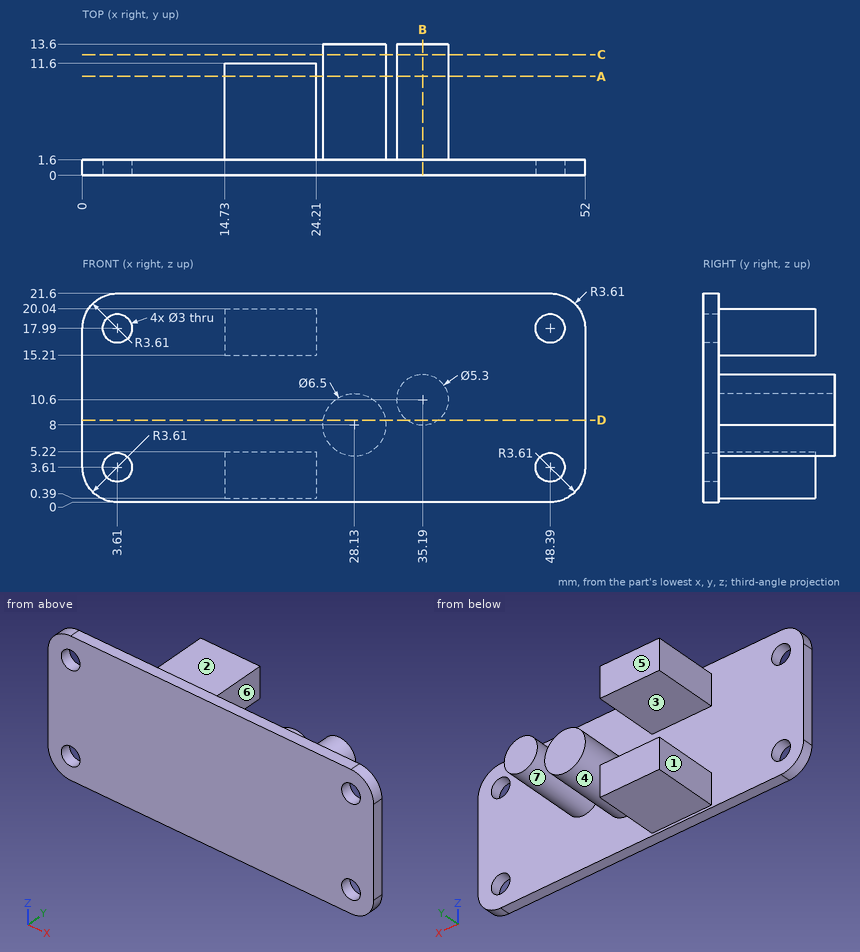
Can you work these out from the drawing? Everything is in mm from the part's minimum corner. A direction names the side the tool comes from. Round coordinates to 2 decimals unless told otherwise and drop trailing zeros. Loops run counter-clockwise (first coordinate to the right, second up) from the corner with the lowest first, then second, coordinate; pieces in that order, holes last. Notation, with made-up numbers: (-2.5, 53) - (13.5, 53) arc R24 ccw to (13.5, 80) - close; hole circle Ø7 at (70, -37). An arc over 180 degrees is marked (long way). Answer in a Markdown table with one row per item. Add a question column.
(1) If we section it at D-D (z = 8.5): Please give me the cut outline in (x, y), plus the area to 3 significant figures.
(2) For the marked faces 1, 2, 3 and 4, which set-ups out of +Z, -Z, +X, -X, +Y, -Y let a thin tool reach every point of the face, with its end or its side?
(3) I need wall thicknesses on line 1 along X through (y, z) = (8, 1.25); line 2 along Y through (x, z) = (26, 12.25); line 3 along Z through (x, y) = (35, 10.5). Which ranges of each line are inside material? Lowest first, please.
(4) If we section it at C-C (y = 12.5): Please give me the cut outline in (x, z).
(5) I'm going to push flat-ended pins straight in: pin 1 (3 mm diameter, centred on x = 19, y = 9, fed in from +Z); pin 2 (1.4 mm diameter, centred on x = 18.5, z = 3, fed in from +Y); pin 3 (3 mm diameter, centred on y = 9, z = 16, fed in from -X). Where does each tip first touch, or does it pass through?
(6) If we mould it in two halves opening along X, with no side actions, what happens to the marked faces 5, 6 and 7? For each: pulls with the +X half, pulls with the -X half, needs draft (parallel to the pull), parting line crosses it, or undercut.
(7) If we section it at A-A (y = 10.25): Please give me the cut outline in (x, z).
(8) If we section it at B-B (x = 35.19): Please give me the cut outline in (y, z), plus the area to 3 significant figures.
Model answer:
| question | item | result |
|---|---|---|
| 1 | outline | (0, 0) - (52, 0) - (52, 1.6) - (36.81, 1.6) - (36.81, 13.6) - (33.57, 13.6) - (33.57, 1.6) - (31.34, 1.6) - (31.34, 13.6) - (24.92, 13.6) - (24.92, 1.6) - (0, 1.6) - close |
| 1 | area | 199 mm² |
| 2 | face 1 | +Z, -Z, -X, +Y |
| 2 | face 2 | +Z, +X, -X, +Y |
| 2 | face 3 | +X, -X, +Y |
| 2 | face 4 | +Y |
| 3 | line 1 | x = 14.73 to 24.21 |
| 3 | line 2 | y = 0 to 1.6 |
| 3 | line 3 | z = 7.96 to 13.24 |
| 4 | outline | circle Ø6.5 at (28.13, 8); circle Ø5.3 at (35.19, 10.6) |
| 5 | pin 1 | stops at z = 20.04 |
| 5 | pin 2 | stops at y = 11.6 |
| 5 | pin 3 | stops at x = 14.73 |
| 6 | face 5 | needs draft |
| 6 | face 6 | pulls with the +X half |
| 6 | face 7 | undercut |
| 7 | outline | (14.73, 0.39) - (24.21, 0.39) - (24.21, 5.22) - (14.73, 5.22) - close; (14.73, 15.21) - (24.21, 15.21) - (24.21, 20.04) - (14.73, 20.04) - close; circle Ø6.5 at (28.13, 8); circle Ø5.3 at (35.19, 10.6) |
| 8 | outline | (0, 0) - (1.6, 0) - (1.6, 7.95) - (13.6, 7.95) - (13.6, 13.25) - (1.6, 13.25) - (1.6, 21.6) - (0, 21.6) - close |
| 8 | area | 98.2 mm² |
